Part model, mm, in its own coordinate system. A direction names the side the tool comes from. Round coordinates to 2 decimals unless told otherwise and drop trailing zeros. Write each loop counter-clockwise with the first axis right and the second up, starting at its lowest first coordinate (ties: lowest second). Pieces come first, ordered by that corner, then holes.
```python
from build123d import *

# Parameters (mm, degrees)
BOSS_EXTRUDE1_DEPTH            = 6.35
BOSS_EXTRUDE2_DEPTH            = 38.1
F_8_CLEARANCE_HOLE1_AT_2_COUNT = 2
F_8_CLEARANCE_HOLE1_AT_2_PITCH = 38.1
CHAMFER1_SIZE                  = 0.254
CHAMFER2_SIZE                  = 0.254


with BuildPart() as part:
    # Sketch1 → Boss-Extrude1 (new body)
    with BuildSketch(Plane(origin=(0, 0, 0), x_dir=(1, 0, 0), z_dir=(0, 1, 0))):
        Polygon((-25.4, 9.525), (-25.4, -9.525), (-12.699999999999996, -9.525), (-12.700000000000003, 9.524999999999993), align=None)
        Polygon((-12.700000000000003, 9.524999999999993), (-12.699999999999996, -9.525), (12.700000000000003, -9.525), (12.700000000000003, 9.524999999999997), align=None)
        Polygon((12.700000000000003, 9.524999999999997), (12.700000000000003, -9.524999999999997), (25.4, -9.525), (25.4, 9.525), align=None)
    extrude(amount=BOSS_EXTRUDE1_DEPTH)

    # Sketch1<3> → Boss-Extrude2 (add)
    with BuildSketch(Plane(origin=(0, 0, 0), x_dir=(1, 0, 0), z_dir=(0, 1, 0))):
        Polygon((-12.700000000000003, 9.524999999999993), (-12.699999999999996, -9.525), (12.700000000000003, -9.525), (12.700000000000003, 9.524999999999997), align=None)
    extrude(amount=BOSS_EXTRUDE2_DEPTH)

    # Sketch4 → 3/8-16 Tapped Hole1 (revolve, cut)
    with BuildSketch(Plane(origin=(0, 25.4, 9.525), x_dir=(0, -1, 0), z_dir=(1, 0, 0))):
        Polygon((0, 0), (-4.67e-15, 19.05), (4.825999999999995, 19.05), (3.9687499999999956, 18.192749999999993), (3.9687499999999973, 0.8572500000000004), (4.826, 0), align=None)
    revolve(axis=Axis((0, 25.4, 15.874999999999991), (0, 0, -1)), mode=Mode.SUBTRACT)

    # Sketch8 → #8 Clearance Hole1 (revolve, cut)
    with BuildSketch(Plane(origin=(-19.05, 6.35, 4.66e-15), x_dir=(0, 0, 1), z_dir=(1, 0, 0))):
        Polygon((0, 0), (-1.56e-15, 6.350000000000001), (2.8828999999999985, 6.350000000000001), (2.247899999999996, 5.714999999999998), (2.247899999999997, 0.6350000000000001), (2.8829, 0), align=None)
    f_8_clearance_hole1 = revolve(axis=Axis((-19.05, 12.69999999999999, 4.66e-15), (0, -1, 0)), mode=Mode.SUBTRACT)

    # #8 Clearance Hole1 at 2: #8 Clearance Hole1 ×2
    with Locations(*[(i * F_8_CLEARANCE_HOLE1_AT_2_PITCH, 0, 0) for i in range(1, F_8_CLEARANCE_HOLE1_AT_2_COUNT)]):
        add(f_8_clearance_hole1, mode=Mode.SUBTRACT)

    # Chamfer1
    chamfer1_edges = [part.edges().sort_by_distance(p)[0] for p in [
        (25.4, 6.35, 0),
        (-19.05, 6.35, -9.525),
        (19.050000000000004, 6.35, 9.525),
        (19.050000000000004, 6.35, -9.525),
        (-25.4, 6.35, 0),
        (0, 38.1, -9.525),
        (-12.7, 38.1, 3.55e-15),
        (3.55e-15, 38.1, 9.525),
        (12.700000000000003, 38.1, 0),
        (-19.049999999999997, 6.35, 9.525),
    ]]
    chamfer(chamfer1_edges, length=CHAMFER1_SIZE)

    # Chamfer2
    chamfer2_edges = [part.edges().sort_by_distance(p)[0] for p in [
        (25.4, 3.048, -9.525),
        (25.4, 3.048, 9.525),
        (-25.4, 3.048, -9.525),
        (-25.4, 3.048, 9.525),
        (-25.4, 0, 0),
        (0, 0, -9.525),
        (25.4, 0, 0),
        (0, 0, 9.525),
        (12.700000000000003, 21.971000000000004, -9.524999999999999),
        (12.700000000000003, 21.971000000000004, 9.524999999999999),
        (-12.699999999999996, 21.971000000000004, 9.525),
        (-12.700000000000003, 21.971000000000004, -9.524999999999999),
    ]]
    chamfer(chamfer2_edges, length=CHAMFER2_SIZE)


solid = part.part
```
Q1. Mould opens along Z. For faces 1 (the flat face through (0, 19, -9.525)), 2 (the flat face through (0, 19, 9.525)), 3 (the cylindrical face through (17.155, 3.211, 1.208)), 4 (the flat face through (-25.4, 3, 0)) say: +Z half, -Z half, draft (parallel to the pull), parting line (faces both ways), or undercut.
Values follow:
face 1: -Z half
face 2: +Z half
face 3: undercut
face 4: draft
Q2. Wall check: L1, parallel to X at y = 4.6, z = 0; L2, parallel to Z at x = -19.05, y = 2.1 (3 decimals); L3, parallel to Y at x = 0, z = 3.5. Give the ranges that are in metal, low to high.
Values follow:
L1: x = -25.4 to -21.3, -16.8 to 16.8, 21.3 to 25.4
L2: z = -9.525 to -2.248, 2.248 to 9.525
L3: y = 0 to 21.43, 29.37 to 38.1
Q3. Cut at A-A on z = 0. State how many separate pieces and enclosed holes the cut face has, plus the area to 3 significant figures.
Values follow:
separate pieces: 3
enclosed holes: 1
area: 1,020 mm2
Q4. Which spindle directions (+Z, -Z, +X, -X, +Y, -Y) get a long thin tool onto all of the face, cutting with end or side? Do faces 5 (the flat face through (25.4, 3, 0)), 6 (the flat face through (12.7, 22, 0)), 7 (the flat face through (-12.7, 22, 0)). Say none if no direction does.
Values follow:
face 5: +Z, -Z, +X, +Y, -Y
face 6: +Z, -Z, +X, +Y
face 7: +Z, -Z, -X, +Y
Q5. Cut at C-C on x = 19.05. Write the cut outline in (y, z) (3 decimals), plus the area to 3 significant figures.
Values follow:
outline: (0, -9.271) - (0.254, -9.525) - (6.096, -9.525) - (6.35, -9.271) - (6.35, -2.883) - (5.715, -2.248) - (0.635, -2.248) - (0, -2.883) - close; (0, 2.883) - (0.635, 2.248) - (5.715, 2.248) - (6.35, 2.883) - (6.35, 9.271) - (6.096, 9.525) - (0.254, 9.525) - (0, 9.271) - close
area: 91.5 mm2
Q6. Drop flat-ended pins along their axis: pin 1 (3.5 mm diameter, centred on x = 18, z = -4, fed in from +Y); pin 2 (3 mm diameter, centred on y = 22.5, z = -4.5, fed in from -X); pin 3 (3.5 mm diameter, centred on x = -19.05, z = 0, fed in from +Y); pin 4 (1 mm diameter, centred on x = -14, z = 1.5, fed in from +Y). Give the stop position or say it passes through.
Values follow:
pin 1: stops at y = 6.35
pin 2: stops at x = -12.7
pin 3: passes through
pin 4: stops at y = 6.35
Q7. Cut at D-D on y = 25.4. Write the cut outline in (x, z) (3 decimals).
Values follow:
outline: (-12.7, -9.271) - (-12.446, -9.525) - (-4.826, -9.525) - (-3.969, -8.668) - (-3.969, 8.668) - (-4.826, 9.525) - (-12.446, 9.525) - (-12.7, 9.271) - close; (3.969, -8.668) - (4.826, -9.525) - (12.446, -9.525) - (12.7, -9.271) - (12.7, 9.271) - (12.446, 9.525) - (4.826, 9.525) - (3.969, 8.668) - close
Q8. Cut at B-B on y = 3.5. Write the cut outline in (x, z) (3 decimals).
Values follow:
outline: (-25.4, -9.271) - (-25.146, -9.525) - (25.146, -9.525) - (25.4, -9.271) - (25.4, 9.271) - (25.146, 9.525) - (-25.146, 9.525) - (-25.4, 9.271) - close; hole circle Ø4.496 at (-19.05, 0); hole circle Ø4.496 at (19.05, 0)
